Work out the finished part from the listing and answer in its coordinate system (mm). A direction names the side the tool comes from. Round coordinates to 2 decimals unless told otherwise and drop trailing zeros. Loops run counter-clockwise (first coordinate to the right, second up) from the corner with the lowest first, then second, coordinate; pieces in that order, holes last. Notation, with made-up numbers: (70.25, 69) - (95.25, 69) arc R20 cw to (95.25, 86) - close; hole circle Ø1 at (64, 40.5). An arc over 180 degrees is marked (long way). Return JSON: item names as keys, results as strings.
Autodesk Inventor part; units mm, degrees
ref_plane "YZ Plane" through (0, 0, 0) normal (1, 0, 0) x (0, 1, 0)
ref_plane "XZ Plane" through (0, 0, 0) normal (0, 1, 0) x (-1, 0, 0)
ref_plane "XY Plane" through (0, 0, 0) normal (0, 0, 1) x (1, 0, 0)
sketch "Sketch1" plane through (0, 0, 0) normal (1, 0, 0) x (0, 1, 0)
  circle A0 centre (0, 0) radius 5
  dimension "d0" = 10
extrude "Extrusion1" add sketch "Sketch1" along normal blind 46
thread "Thread1"
chamfer "Chamfer1" distance 1 angle 45 1 edges at (46, -5, 0)
sketch "Sketch2" plane through (46, 0, 0) normal (1, 0, 0) x (0, 0, -1)
  circle A0 centre (0, 0) radius 3
  dimension "d8" = 6
extrude "Extrusion2" add sketch "Sketch2" along normal blind 14
sketch "Sketch3" plane through (60, 0, 0) normal (1, 0, 0) x (0, 0, -1)
  circle A0 centre (0, 0) radius 2.5
  line L0 (-1.7349, 1.8) -> (1.7349, 1.8)
  dimension "d11" = 5
  dimension "d12" = 1.8
extrude "Extrusion3" add sketch "Sketch3" along normal blind 10 contours A0 L0 picked at (0.076, 0.3701)
mirror "Mirror1" about plane through (0, 0, 0) normal (-1, 0, 0) of "Extrusion1", "Chamfer1", "Extrusion2", "Extrusion3"
properties part number "КВ33.000.104 - Вал" material "Iron, Ductile"
1) Section B-B (z = 0) is taken. Give the vertices of the cut face in (x, y), and give its area (3 significant figures).
Verdict:
{"outline": "(-70, -2.5) - (-60, -2.5) - (-60, -3) - (-46, -3) - (-46, -4) - (-45, -5) - (45, -5) - (46, -4) - (46, -3) - (60, -3) - (60, -2.5) - (70, -2.5) - (70, 1.8) - (60, 1.8) - (60, 3) - (46, 3) - (46, 4) - (45, 5) - (-45, 5) - (-46, 4) - (-46, 3) - (-60, 3) - (-60, 1.8) - (-70, 1.8) - close", "area": "1,170 mm2"}
2) Flat-ended cylindrical pins translate along their axes: pin 1 (5 mm diameter, centred on y = 3.5, z = 4, fed in from -X); pin 2 (2 mm diameter, centred on x = 10, y = 2.5, fed in from +Z); pin 3 (3 mm diameter, centred on x = -66.5, z = -1, fed in from +Y). Find the tip coordinate at first contact, or state that the pin passes through.
Verdict:
{"pin 1": "stops at x = -60", "pin 2": "stops at z = 4.77", "pin 3": "stops at y = 1.8"}
3) Section C-C (x = -43.5) is taken. Give the vertices of the cut face in (y, z).
Verdict:
{"outline": "circle Ø10 at (0, 0)"}
4) Section A-A (y = 0) is taken. Give the vertices of the cut face in (x, z), and give its area (3 significant figures).
Verdict:
{"outline": "(-70, -2.5) - (-60, -2.5) - (-60, -3) - (-46, -3) - (-46, -4) - (-45, -5) - (45, -5) - (46, -4) - (46, -3) - (60, -3) - (60, -2.5) - (70, -2.5) - (70, 2.5) - (60, 2.5) - (60, 3) - (46, 3) - (46, 4) - (45, 5) - (-45, 5) - (-46, 4) - (-46, 3) - (-60, 3) - (-60, 2.5) - (-70, 2.5) - close", "area": "1,190 mm2"}
5) Find the intervals of material crossed by L1, parallel to Z at x = -40.5, y = 3; L2, parallel to Z at x = 6, y = -0.25; L3, parallel to X at y = 1.25, z = -2.25, in increasing order.
Verdict:
{"L1": "z = -4 to 4", "L2": "z = -4.99 to 4.99", "L3": "x = -60 to 60"}
6) A tool of negligible diameter and unlimited length cuts with its end or side. For faces 1 (the flat face through (-65, 1.8, 0)), 2 (the cylindrical face through (64.9, -2.5, -0.1)), 3 (the cylindrical face through (-64.9, -2.5, 0.1)), 4 (the flat face through (-70, 0, 0)), 5 (the flat face through (65, 1.8, 0)), from which of +Z, -Z, +X, -X, +Y, -Y can it reach the whole face along a straight path? Write none if from no direction.
Verdict:
{"face 1": "+Z, -Z, -X, +Y", "face 2": "+X", "face 3": "-X", "face 4": "+Z, -Z, -X, +Y, -Y", "face 5": "+Z, -Z, +X, +Y"}
